```python
from build123d import *

# Parameters (mm, degrees)
EXTRUDE_1_DEPTH       = 244
EXTRUDE_3_DEPTH       = 244
PATTERN_CURVE_1_COUNT = 11
PATTERN_CURVE_1_PITCH = 10
SKETCH_3_R            = 2.25
CUT_EXTRUDE_1_DEPTH   = 6
SKETCH_4_R            = 1.25
SKETCH_4_R_2          = 1.6
CUT_EXTRUDE_2_DEPTH   = 5.5
SKETCH_5_R            = 2.1
SKETCH_5_R_2          = 1.6
CUT_EXTRUDE_3_DEPTH   = 6


with BuildPart() as part:
    # Эскиз1 → Вытянуть1 (new body)
    with BuildSketch(Plane.XY):
        with BuildLine():
            Line((0, 40), (1.528979332, 40))
            ThreePointArc((1.528979332, 40), (2.225614441, 39.717425624), (2.528547087, 39.029399052))
            Line((2.528547087, 39.029399052), (3.5, 6))
            Line((3.5, 6), (118.5, 6))
            Line((118.5, 6), (119.471452913, 39.029399052))
            ThreePointArc((119.471452913, 39.029399052), (119.774385559, 39.717425624), (120.471020668, 40))
            Line((120.471020668, 40), (122, 40))
            Line((122, 40), (122, 0))
            Line((122, 0), (0, 0))
            Line((0, 0), (0, 40))
        make_face()
    extrude(amount=EXTRUDE_1_DEPTH)

    # Эскиз2 → Вытянуть3 (add)
    with BuildSketch(Plane.XY.offset(244)):
        with BuildLine():
            Line((10.5, 39.5), (9.25, 6))
            Line((9.25, 6), (12.75, 6))
            Line((12.75, 6), (11.5, 39.5))
            ThreePointArc((11.5, 39.5), (11, 40), (10.5, 39.5))
        make_face()
    extrude_3 = extrude(amount=-EXTRUDE_3_DEPTH)

    # Кривая1: Вытянуть3 ×11
    with Locations(*[(i * PATTERN_CURVE_1_PITCH, 0, 0) for i in range(1, PATTERN_CURVE_1_COUNT)]):
        add(extrude_3)

    # Эскиз3 → Вырез-Вытянуть1 (cut)
    with BuildSketch(Plane.XZ):
        with Locations((26, 236)):
            Circle(SKETCH_3_R)
        with Locations((96, 236)):
            Circle(SKETCH_3_R)
        with Locations(Location((96, 8, 0), (0, 0, 180))):
            Circle(SKETCH_3_R)
        with Locations(Location((26, 8, 0), (0, 0, 180))):
            Circle(SKETCH_3_R)
    extrude(amount=-CUT_EXTRUDE_1_DEPTH, mode=Mode.SUBTRACT)

    # Эскиз4 → Вырез-Вытянуть2 (cut)
    with BuildSketch(Plane(origin=(-5.723570629, 0, -26.359021189), x_dir=(1, 0, 0), z_dir=(0, -1, 0))):
        with Locations((75.723570629, 72.359021189)):
            Circle(SKETCH_4_R)
        with Locations((90.223570629, 189.359021189)):
            Circle(SKETCH_4_R_2)
        with Locations((90.223570629, 49.359021189)):
            Circle(SKETCH_4_R_2)
        with Locations((57.223570629, 147.359021189)):
            Circle(SKETCH_4_R_2)
        with Locations((57.223570629, 128.359021189)):
            Circle(SKETCH_4_R_2)
        with Locations((75.723570629, 46.359021189)):
            Circle(SKETCH_4_R)
        with Locations((57.223570629, 116.359021189)):
            Circle(SKETCH_4_R_2)
        with Locations((57.223570629, 69.859021189)):
            Circle(SKETCH_4_R_2)
    extrude(amount=-CUT_EXTRUDE_2_DEPTH, mode=Mode.SUBTRACT)

    # Эскиз5 → Вырез-Вытянуть3 (cut)
    with BuildSketch(Plane(origin=(128.324191418, 0, 423.775874855), x_dir=(-1, 0, 0), z_dir=(0, -1, 0))):
        with Locations(Location((81.324191418, 273.775874855, 0), (0, 0, 180))):
            Circle(SKETCH_5_R)
        with Locations((21.324191418, 239.775874855)):
            Circle(SKETCH_5_R_2)
        with Locations((81.324191418, 239.775874855)):
            Circle(SKETCH_5_R_2)
        with Locations(Location((81.324191418, 204.775874855, 0), (0, 0, 180))):
            Circle(SKETCH_5_R_2)
        with Locations(Location((21.324191418, 204.775874855, 0), (0, 0, 180))):
            Circle(SKETCH_5_R_2)
    extrude(amount=-CUT_EXTRUDE_3_DEPTH, mode=Mode.SUBTRACT)


solid = part.part
```
Here's how the part is built. I have some questions about the finished solid (model axes, mm). A direction names the side the tool comes from. Coordinates: 2 decimals unless noted, no trailing zeros. One line per question, with ' | ' between items. Start each with the question number.
1. If we section it at A-A (y = 10.5): Give the number of separate pieces and of enclosed holes in the cut face, and give its area (3 significant figures).
2. I'm going to push flat-ended pins straight in: pin 1 Ø3 at (x, z) = (51.5, 90) entering from -Y; pin 2 Ø5 at (x, z) = (26.5, 63) entering from +Y; pin 3 Ø1.5 at (x, z) = (70, 46) entering from +Y; pin 4 Ø2.5 at (x, z) = (107, 184) entering from +Y. Where does each tip first touch, or does it pass through?
3. If we mould it in two halves opening along X, with no side actions, what happens to faces 3 (the flat face through (112.134, 22.516, 123.708)), 4 (the flat face through (61, 13, 0)), 5 (the flat face through (0, 20, 120))? For each: released by +X, released by -X, zero draft, split by the parting line, or undercut.
4. Please list where these lines run through material, in increasing order: line 1 along Z through (x, y) = (107, 3.4); line 2 along Z through (x, y) = (47, 3); line 3 along Z through (x, y) = (26, 1.3). Write a range as [from, to].
5. Which directions (+Z, -Z, +X, -X, +Y, -Y) give clear straight access to the entire face, cutting with the end or side of a thin tool? Please do faces 1 (the flat face through (62, 0, 120)), 2 (the flat face through (106, 6, 120)).
Model answer:
1) separate pieces: 13 | enclosed holes: 0 | area: 10,100 mm²
2) pin 1: stops at y = 5.5 | pin 2: stops at y = 6 | pin 3: stops at y = 39.93 | pin 4: passes through
3) face 3: undercut | face 4: zero draft | face 5: released by -X
4) line 1: z = [0, 182.4], [185.6, 217.4], [220.6, 244] | line 2: z = [0, 147.9], [152.1, 182.4], [185.6, 217.4], [220.6, 244] | line 3: z = [0, 5.75], [10.25, 233.75], [238.25, 244]
5) face 1: +Z, -Z, +X, -X, -Y | face 2: +Z, -Z, +Y
